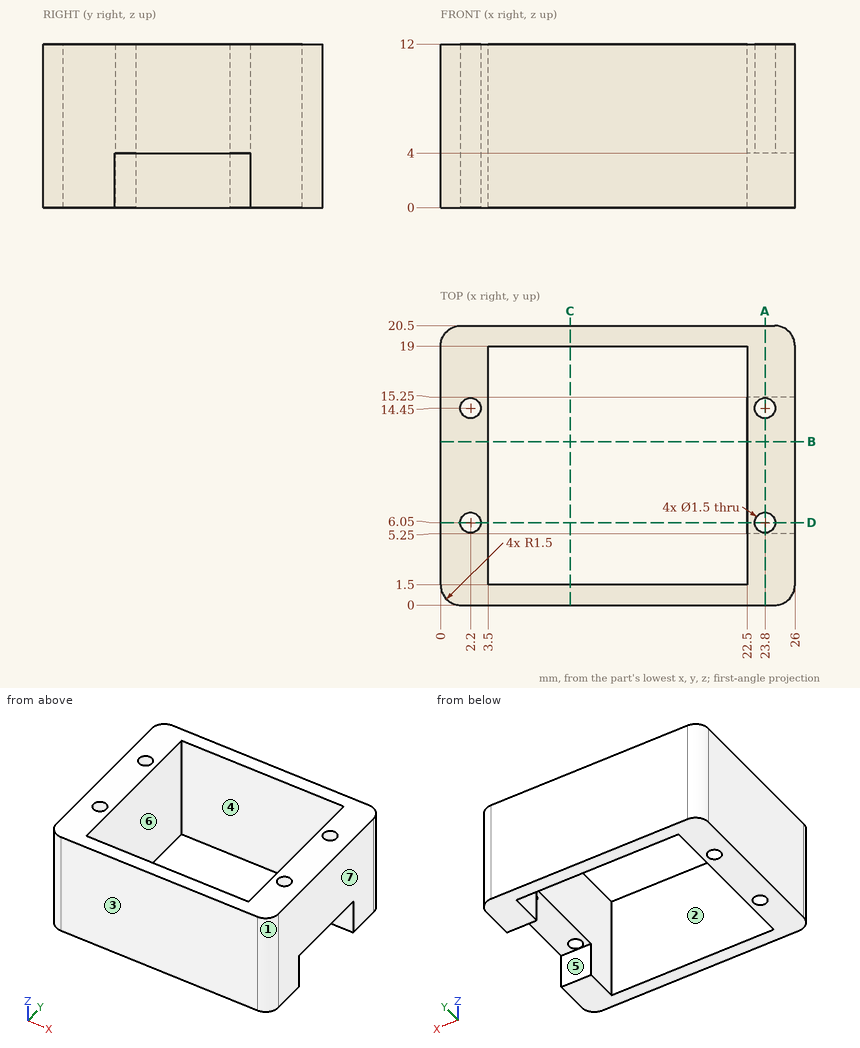
Verification items for this drawing (mm, ordinates from the low corner). A direction names the side the tool comes from. Coordinates: 2 decimals unless noted, no trailing zeros. Loops run counter-clockwise (first coordinate to the right, second up) from the corner with the lowest first, then second, coordinate; pieces in that order, holes last.
Item 1: Sectioned sample at C-C, the plane x = 9.5. Record the boundary of the cut face in (y, z), then the cut area to 3 significant figures.
Item 2: Sectioned sample at A-A, the plane x = 23.8. Record the boundary of the cut face in (y, z), then the cut area to 3 significant figures.
Item 3: Sectioned sample at D-D, the plane y = 6.05. Record the boundary of the cut face in (x, z), then the cut area to 3 significant figures.
Item 4: Access from +Z, -Z, +X, -X, +Y, -Y to the whole of each face (thin tool, end or side, straight path). Record for the marked faces 5, 6 and 7.
Item 5: Thickness scan on line 1 (Y direction, x = 23.8, z = 10.25); line 2 (X direction, y = 6, z = 11.5); line 3 (X direction, y = 2.5, z = 4.25). Record the ranges inside material, lowest first.
Item 6: Go/stop test with flat-tipped pins: pin 1 Ø3 at (x, y) = (24.5, 10) entering from -Z; pin 2 Ø1.2 at (x, y) = (23.8, 14.45) entering from +Z. Record where each tip stops, or that it passes through.
Item 7: Release check for a two-part mould opening along X. For the marked faces 1, 2, 3 and 4 record: released by +X, released by -X, zero draft, split by the parting line, or undercut.
Item 8: Sectioned sample at B-B, the plane y = 12. Record the boundary of the cut face in (x, z), then the cut area to 3 significant figures.
Check result:
1. outline: (0, 0) - (1.5, 0) - (1.5, 12) - (0, 12) - close; (19, 0) - (20.5, 0) - (20.5, 12) - (19, 12) - close
1. area: 36.0 mm2
2. outline: (0, 0) - (5.25, 0) - (5.25, 4) - (5.3, 4) - (5.3, 12) - (0, 12) - close; (6.8, 4) - (13.7, 4) - (13.7, 12) - (6.8, 12) - close; (15.2, 4) - (15.25, 4) - (15.25, 0) - (20.5, 0) - (20.5, 12) - (15.2, 12) - close
2. area: 182 mm2
3. outline: (0, 0) - (1.45, 0) - (1.45, 12) - (0, 12) - close; (2.95, 0) - (3.5, 0) - (3.5, 12) - (2.95, 12) - close; (22.5, 4) - (23.05, 4) - (23.05, 12) - (22.5, 12) - close; (24.55, 4) - (26, 4) - (26, 12) - (24.55, 12) - close
3. area: 40.0 mm2
4. face 5: -Z, +X
4. face 6: +Z, -Z
4. face 7: +Z, -Z, +X, +Y, -Y
5. line 1: y = 0 to 5.3, 6.8 to 13.7, 15.2 to 20.5
5. line 2: x = 0 to 1.45, 2.95 to 3.5, 22.5 to 23.05, 24.55 to 26
5. line 3: x = 0 to 3.5, 22.5 to 26
6. pin 1: stops at z = 4
6. pin 2: passes through
7. face 1: released by +X
7. face 2: undercut
7. face 3: zero draft
7. face 4: undercut
8. outline: (0, 0) - (3.5, 0) - (3.5, 12) - (0, 12) - close; (22.5, 4) - (26, 4) - (26, 12) - (22.5, 12) - close
8. area: 70.0 mm2
